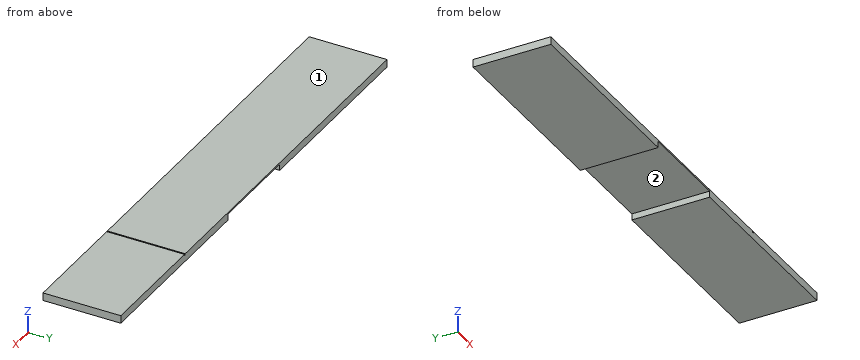
```python
from build123d import *

# Parameters (mm, degrees)
F1_DEPTH = 25
F2_W     = 0.4
F2_H     = 25
F3_DEPTH = 0.5


with BuildPart() as f1:
    # F0 (on Front) → F1 (new body)
    with BuildSketch(Plane.XZ):
        Polygon((77.5, 0), (-77.5, 0), (-77.5, -2.5), (-15, -2.5), (-15, -0.5), (15, -0.5), (15, -2.5), (77.5, -2.5), align=None)
    extrude(amount=F1_DEPTH)

    # F2 (on face) → F3 (cut, through all)
    with BuildSketch(Plane.XY):
        with Locations((40.2, -12.5)):
            Rectangle(F2_W, F2_H)
    extrude(amount=-F3_DEPTH, mode=Mode.SUBTRACT)


solid = f1.part
```
For this review, take the finished solid that the model builds, in its own axes (mm). Face numbers are marked on the shaded views. A direction names the side the tool comes from. Coordinates: 2 decimals unless noted, no trailing zeros. Order: outer loops, then holes, each group sorted by start corner. A loop starts at its lowest first (then second) coordinate and runs counter-clockwise, first axis right, second up. Notation, with made-up numbers: (3, 2) -> (8, 2) arc R24 cw to (8, 17) -> close; hole circle Ø3 at (-31.5, 84.25). An arc over 180 degrees is marked (long way). Use CSV: the item, a comma, the result in double quotes. Start each with the question number.
Item 1: Wall thickness on probe 1 along X at (y, z) = (-5, -2.15); probe 2 along X at (y, z) = (-10.5, -0.1); probe 3 along Z at (x, y) = (-10, -4): over which ranges is each line inside the solid? List them lowest first.
Item 2: For the marked faces 1 and 2, list the 3-axis set-ups (+Z, -Z, +X, -X, +Y, -Y) from which the entire face can be reached by the end or side of a thin tool; tool diameter is ignored.
Item 3: Insertion check: pin 1 (12.5 mm diameter, centred on x = 5, y = -12.5, fed in from -Z). The pin has a flat end and moves straight along its axis. Give the tip position at first contact, or say it passes through.
Item 4: We need section C-C, the plane x = -9.5. Give the boundary of the cut face in (y, z).
Item 5: We need section B-B, the plane y = -9.75. Give the boundary of the cut face in (x, z).
Item 6: We need section A-A, the plane z = -1.7. Give the boundary of the cut face in (x, y).
Derived:
1,probe 1,"x = -77.5 to -15, 15 to 77.5"
1,probe 2,"x = -77.5 to 40, 40.4 to 77.5"
1,probe 3,"z = -0.5 to 0"
2,face 1,"+Z, +X, -X, +Y, -Y"
2,face 2,"-Z, +Y, -Y"
3,pin 1,"stops at z = -0.5"
4,outline,"(-25, -0.5) -> (0, -0.5) -> (0, 0) -> (-25, 0) -> close"
5,outline,"(-77.5, -2.5) -> (-15, -2.5) -> (-15, -0.5) -> (15, -0.5) -> (15, -2.5) -> (77.5, -2.5) -> (77.5, 0) -> (40.4, 0) -> (40.4, -0.5) -> (40, -0.5) -> (40, 0) -> (-77.5, 0) -> close"
6,outline,"(-77.5, -25) -> (-15, -25) -> (-15, 0) -> (-77.5, 0) -> close; (15, -25) -> (77.5, -25) -> (77.5, 0) -> (15, 0) -> close"
